Geometry check sheet. Reference: the model listing, model coordinates, mm. A direction names the side the tool comes from. Round coordinates to 2 decimals unless told otherwise and drop trailing zeros. Write each loop counter-clockwise with the first axis right and the second up, starting at its lowest first coordinate (ties: lowest second). Pieces come first, ordered by that corner, then holes. Notation, with made-up numbers: (68, -14) - (92, -14) arc R8 cw to (92, -2) - close; hole circle Ø2 at (-30.75, 24.25). An arc over 180 degrees is marked (long way). Return JSON: item names as keys, results as strings. Group by question number.
from build123d import *

# Parameters (mm, degrees)
F0_W     = 6
F0_H     = 0.3
F1_DEPTH = 2.5
F2_R     = 2


# Not quite as in the source:
# - a feature names something its author has since deleted; it is built from what else it names


with BuildPart() as f1:
    # F0 (on Top) → F1 (new body)
    with BuildSketch(Plane.XY):
        Polygon((0, -4), (-3.5, -0.5), (-3.5, -65.5), (-23.5, -65.5), (-23.5, -70.5), (-17.5, -70.5), (-1.25, -70.5), (-1.25, -55.5), (1.25, -55.5), (1.25, -70.5), (17.5, -70.5), (23.5, -70.5), (23.5, -65.5), (3.5, -65.5), (3.5, -0.5), align=None)
        with Locations((-20.5, -70.65)):
            Rectangle(F0_W, F0_H)
        with Locations((20.5, -70.65)):
            Rectangle(F0_W, F0_H)
        Polygon((-20, 16), (-3.5, -0.5), (0, -4), (3.5, -0.5), (20, 16), (0, 36), align=None)
    extrude(amount=F1_DEPTH)

    # F2
    f2_edges = [f1.edges().sort_by_distance(p)[0] for p in [
        (3.5, -65.5, 1.25),
        (-3.5, -65.5, 1.25),
        (-23.5, -65.5, 1.25),
        (23.5, -65.5, 1.25),
        (-23.5, -70.8, 1.25),
        (23.5, -70.8, 1.25),
        (20, 16, 1.25),
        (0, 36, 1.25),
        (-20, 16, 1.25),
        (3.5, -0.5, 1.25),
        (-3.5, -0.5, 1.25),
    ]]
    fillet(f2_edges, radius=F2_R)


solid = f1.part
1. Section check A-A (x = -10.5). Enter the section's corners in (y, z).
2. Depth check by flat-ended pin: pin 1 Ø0.8 at (y, z) = (-65.5, 1) entering from +X; pin 2 Ø1.2 at (x, z) = (15, 1.5) entering from +Y; pin 3 Ø1 at (y, z) = (-21, 1) entering from +X. Enter the tip coordinate at first touch or a pass-through.
3. Mould release check, pull along X, two halves, no side actions. Record for faces 4 (the face through (-22.9, -66.07, 1.27)), 5 (the face through (-9, -70.5, 1)), 6 (the face through (4.1, -64.93, 1.27)): pulls with the +X half, pulls with the -X half, needs draft (parallel to the pull), parting line crosses it, or undercut.
4. Tool access check on faces 1 (the face through (-4.07, -64.9, 1.27)), 2 (the face through (9, -70.5, 1)), 3 (the face through (14, -65.5, 1)). Record the directions out of +Z, -Z, +X, -X, +Y, -Y that give a thin tool (end or side, any length) a straight path to the whole face; none if there is none.
5. Material ranges on line 1 along X through (y, z) = (-20.5, 2.2); line 2 along X through (y, z) = (-58, 1.7); line 3 along Y through (x, z) = (-4, 1.6), recorded low to high.
6. Section check B-B (x = 7). Enter the section's corners in (y, z), and give its area (3 significant figures).
7. Section check D-D (y = 20). Enter the section's corners in (x, z), and give its area (3 significant figures).
Result sheet:
{
 "1": {"outline": "(-70.5, 0) - (-65.5, 0) - (-65.5, 2.5) - (-70.5, 2.5) - close; (6.5, 0) - (25.5, 0) - (25.5, 2.5) - (6.5, 2.5) - close"},
 "2": {"pin 1": "stops at x = 22.7", "pin 2": "stops at y = 21.6", "pin 3": "stops at x = 3.5"},
 "3": {"face 4": "pulls with the -X half", "face 5": "undercut", "face 6": "pulls with the +X half"},
 "4": {"face 1": "+Z, -Z, -X", "face 2": "+Z, -Z, -Y", "face 3": "+Z, -Z, +X"},
 "5": {"line 1": "x = -3.5 to 3.5", "line 2": "x = -3.5 to -1.25, 1.25 to 3.5", "line 3": "y = -70.5 to -64.82, -0.01 to 32"},
 "6": {"outline": "(-70.5, 0) - (-65.5, 0) - (-65.5, 2.5) - (-70.5, 2.5) - close; (3, 0) - (29, 0) - (29, 2.5) - (3, 2.5) - close", "area": "77.5 mm²"},
 "7": {"outline": "(-16, 0) - (16, 0) - (16, 2.5) - (-16, 2.5) - close", "area": "80.0 mm²"}
}
